Could you check a few things on this model? Use its own coordinates, in mm. A direction names the side the tool comes from. Round coordinates to 2 decimals unless told otherwise and drop trailing zeros. Loops run counter-clockwise (first coordinate to the right, second up) from the corner with the lowest first, then second, coordinate; pieces in that order, holes last. Notation, with made-up numbers: (-12.5, 43) -> (30.5, 43) arc R19 cw to (30.5, 76) -> close; hole circle Ø1 at (-5, 4). An arc over 180 degrees is marked (long way). One line per item, written item: value.
from build123d import *

# Parameters (mm, degrees)
SKETCH2_R           = 10.5
SKETCH2_R_2         = 5.5
BOSS_EXTRUDE1_DEPTH = 180
SKETCH6_W           = 180
SKETCH6_H           = 70
BOSS_EXTRUDE2_DEPTH = 4
SKETCH8_W           = 180
SKETCH8_H           = 70
SKETCH8_W_2         = 170
SKETCH8_H_2         = 60
BOSS_EXTRUDE3_DEPTH = 55
SKETCH9_W           = 15
SKETCH9_H           = 7
CUT_EXTRUDE1_DEPTH  = 5
SKETCH10_W          = 14
SKETCH10_H          = 8
CUT_EXTRUDE2_DEPTH  = 5
SKETCH11_R          = 4
CUT_EXTRUDE3_DEPTH  = 2


with BuildPart() as part:
    # Sketch2 → Boss-Extrude1 (new body)
    with BuildSketch(Plane(origin=(0, 0, 0), x_dir=(0, 0, -1), z_dir=(1, 0, 0))):
        with Locations(Location((0, 0, 0), (0, 0, 180))):
            Circle(SKETCH2_R)
        with Locations(Location((0, 0, 0), (0, 0, 180))):
            Circle(SKETCH2_R_2, mode=Mode.SUBTRACT)
    extrude(amount=BOSS_EXTRUDE1_DEPTH)

    # Sketch6 → Boss-Extrude2 (add)
    with BuildSketch(Plane(origin=(0, 10, 0), x_dir=(1, 0, 0), z_dir=(0, 1, 0))):
        with Locations((90.013629188, 0)):
            Rectangle(SKETCH6_W, SKETCH6_H)
    extrude(amount=-BOSS_EXTRUDE2_DEPTH)

    # Sketch8 → Boss-Extrude3 (add)
    with BuildSketch(Plane(origin=(0, 10, 0), x_dir=(1, 0, 0), z_dir=(0, 1, 0))):
        with Locations((90.013629188, 0)):
            Rectangle(SKETCH8_W, SKETCH8_H)
        with Locations((90.013629188, 0)):
            Rectangle(SKETCH8_W_2, SKETCH8_H_2, mode=Mode.SUBTRACT)
    extrude(amount=BOSS_EXTRUDE3_DEPTH)

    # Sketch9 → Cut-Extrude1 (cut)
    with BuildSketch(Plane(origin=(180.013629188, 0, 0), x_dir=(0, 0, -1), z_dir=(1, 0, 0))):
        with Locations((0, 27.5)):
            Rectangle(SKETCH9_W, SKETCH9_H)
    extrude(amount=-CUT_EXTRUDE1_DEPTH, mode=Mode.SUBTRACT)

    # Sketch10 → Cut-Extrude2 (cut)
    with BuildSketch(Plane.ZY.offset(-0.013629188)):
        with Locations((0, 26)):
            Rectangle(SKETCH10_W, SKETCH10_H)
    extrude(amount=-CUT_EXTRUDE2_DEPTH, mode=Mode.SUBTRACT)

    # Sketch11 → Cut-Extrude3 (cut)
    with BuildSketch(Plane(origin=(0, 65, 0), x_dir=(1, 0, 0), z_dir=(0, 1, 0))):
        with Locations((5.013629188, 30)):
            Circle(SKETCH11_R)
        with Locations((175.656317999, 30)):
            Circle(SKETCH11_R)
        with Locations((5.013629188, -30)):
            Circle(SKETCH11_R)
        with Locations((175.013629188, -30)):
            Circle(SKETCH11_R)
    extrude(amount=-CUT_EXTRUDE3_DEPTH, mode=Mode.SUBTRACT)


solid = part.part
(1) If we section it at C-C, the plane y = 13.5: Please give me the cut outline in (x, z), then the cut area to 3 significant figures.
Recorded:
outline: (0.01, -35) -> (180.01, -35) -> (180.01, 35) -> (0.01, 35) -> close; hole (5.01, -30) -> (175.01, -30) -> (175.01, 30) -> (5.01, 30) -> close
area: 2,400 mm²
(2) If I drill on L1, parallel to Z at x = 54.5, y = 46.5; L2, parallel to X at y = 36, z = 28; L3, parallel to Y at x = 108.5, z = 0, over which ranges is the centre line in solid material (lowest first)?
Recorded:
L1: -35 to -30, 30 to 35
L2: 0.01 to 5.01, 175.01 to 180.01
L3: -10.5 to -5.5, 5.5 to 10.5
(3) If we section it at B-B, the plane z = 0: Give the number of separate pieces and of enclosed holes in the cut face, then the cut area to 3 significant figures.
Recorded:
separate pieces: 4
enclosed holes: 0
area: 2,270 mm²
(4) If we section it at D-D, the plane z = -24: Please give me the cut outline in (x, y).
Recorded:
outline: (0.01, 6) -> (180.01, 6) -> (180.01, 65) -> (175.01, 65) -> (175.01, 10) -> (5.01, 10) -> (5.01, 65) -> (0.01, 65) -> close
(5) Thinking about a two-plate mould opening in X: for faces 6 (the face through (178, 31, 0)), 7 (the face through (175.014, 37, 0)), 8 (the face through (0.014, 35, 0)), 9 (the face through (88.8, 10.5, 0)), which applies, released by +X, released by -X, zero draft, split by the parting line, or undercut?
Recorded:
face 6: zero draft
face 7: undercut
face 8: released by -X
face 9: undercut
(6) I'm going to push flat-ended pins straight in: pin 1 Ø8.5 at (y, z) = (-2, 3) entering from +X; pin 2 Ø12 at (x, z) = (159, 11) entering from -Y; pin 3 Ø1 at (x, z) = (29.5, -10) entering from -Y; pin 4 Ø6.5 at (x, z) = (177.5, -28.5) entering from +Y. Where does each tip first touch, or does it pass through?
Recorded:
pin 1: x = 180
pin 2: y = -9.23
pin 3: y = -4.47
pin 4: y = 65
(7) For faces 1 (the face through (4, 63, 31)), 2 (the face through (178, 27, -7.5)), 3 (the face through (0, 5, 5)), 4 (the face through (2, 30, 0)), 5 (the face through (2, 26, 7)), which set-ups out of +Z, -Z, +X, -X, +Y, -Y let a thin tool reach every point of the face, with its end or its side?
Recorded:
face 1: +Y
face 2: +X
face 3: +Z, -Z, -X, +Y, -Y
face 4: +X, -X
face 5: -X
(8) If we section it at A-A, the plane y = 0: Please give me the cut outline in (x, z), then the cut area to 3 significant figures.
Recorded:
outline: (0, -10.5) -> (180, -10.5) -> (180, -5.5) -> (0, -5.5) -> close; (0, 5.5) -> (180, 5.5) -> (180, 10.5) -> (0, 10.5) -> close
area: 1,800 mm²
